```python
from build123d import *

# Parameters (mm, degrees)
BOSS_EXTRUDE1_DEPTH = 10.4
CIRPATTERN1_COUNT   = 10
BOSS_EXTRUDE2_START = 2
SKETCH2_R           = 20
SKETCH2_R_2         = 10.5
BOSS_EXTRUDE2_DEPTH = 2


with BuildPart() as part:
    # Sketch1 → Boss-Extrude1 (new body)
    with BuildSketch(Plane.XY):
        with BuildLine():
            ThreePointArc((9.845402976, 13.551034656), (5.176034656, 15.930196648), (0, 16.75))
            Line((0, 16.75), (1.800167381, 14.035023954))
            ThreePointArc((1.800167381, 14.035023954), (2.401185606, 12.498693353), (3.754556503, 11.555336666))
            ThreePointArc((3.754556503, 11.555336666), (5.403947685, 11.523036823), (6.793214092, 12.412684734))
            Line((6.793214092, 12.412684734), (9.845402976, 13.551034656))
        make_face()
        with BuildLine():
            Line((0, 20), (0, 16.75))
            ThreePointArc((0, 16.75), (5.176034656, 15.930196648), (9.845402976, 13.551034656))
            Line((9.845402976, 13.551034656), (11.755705046, 16.180339887))
            ThreePointArc((11.755705046, 16.180339887), (6.180339887, 19.021130326), (0, 20))
        make_face()
    boss_extrude1 = extrude(amount=BOSS_EXTRUDE1_DEPTH)

    # CirPattern1: Boss-Extrude1 ×10 about axis
    cirpattern1_axis = Axis((0, 0, 0), (0, 0, 1))
    for i in range(1, CIRPATTERN1_COUNT):
        add(boss_extrude1.rotate(cirpattern1_axis, i * 360 / CIRPATTERN1_COUNT))

    # Sketch2 → Boss-Extrude2 (add)
    with BuildSketch(Plane(origin=(0, 0, 0), x_dir=(-1, 0, 0), z_dir=(0, 0, -1)).offset(BOSS_EXTRUDE2_START)):
        Circle(SKETCH2_R)
        Circle(SKETCH2_R_2, mode=Mode.SUBTRACT)
    extrude(amount=-BOSS_EXTRUDE2_DEPTH)


solid = part.part
```
Design review of the part built by this model. Coordinates are the model's own, in mm. A direction names the side the tool comes from. Give positions to 0.01 mm unless a question says otherwise; leave off trailing zeros. Loops run counter-clockwise (first coordinate to the right, second up) from the corner with the lowest first, then second, coordinate; pieces in that order, holes last. Notation, with made-up numbers: M 22.5,-32.5 L 74.5,-32.5 A5 ccw 74.5,-27.5 Z; hole C 85,45.25 d8. An arc over 180 degrees is marked long. Return JSON: item names as keys, results as strings. Group by question number.
Item 1: Insertion check: pin 1 Ø2 at (y, z) = (-14, 4) entering from +X; pin 2 Ø9.5 at (x, y) = (1.5, 2.5) entering from +Z; pin 3 Ø5 at (y, z) = (3, 0) entering from +X; pin 4 Ø1 at (y, z) = (12.5, 5) entering from +X. Each pin has a flat end and moves straight along its axis. Give the tip position at first contact, or say it passes through.
Item 2: Mouldability with a two-part tool opening along X and no side actions: class faces 1 (the flat face through (8.34, -12.99, 5.13)), 2 (the flat face through (-9, -9, -2)) as released by +X, released by -X, zero draft, split by the parting line, or undercut.
Item 3: We need section A-A (y = 1.5). Give the boundary of the cut face in (x, z), and give its area (3 significant figures).
Item 4: For probe 1 along Y at (x, z) = (0, -1.4); probe 2 along Y at (x, z) = (14, 7); probe 3 along Y at (x, z) = (-13, 3.75), list the stretches that pass through material, from the lowest coordinate up.
Item 5: We need section B-B (y = 18.5). Give the boundary of the cut face in (x, z).
Item 6: Tool access review of faces 3 (the flat face through (-0.89, -15.41, 5.13)), 4 (the cylindrical face through (-10, 3.2, -1)): name each direction out of +Z, -Z, +X, -X, +Y, -Y from which nothing blocks a thin tool from reaching the whole face with its end or side.
Output:
{
 "1": {"pin 1": "stops at x = 15.2", "pin 2": "passes through", "pin 3": "stops at x = 19.99", "pin 4": "stops at x = 16"},
 "2": {"face 1": "undercut", "face 2": "zero draft"},
 "3": {"outline": "M -19.94,-2 L -10.39,-2 L -10.39,0 L -12.58,0 L -12.58,10.4 L -19.94,10.4 Z; M 10.39,-2 L 19.94,-2 L 19.94,10.4 L 12.58,10.4 L 12.58,0 L 10.39,0 Z", "area": "191 mm^2"},
 "4": {"probe 1": "y = -20 to -10.5, 10.5 to 20", "probe 2": "y = -14.28 to -5.71, -2.75 to 2.75, 5.71 to 14.28", "probe 3": "y = -15.2 to -5.99, -2.03 to 2.03, 5.99 to 15.2"},
 "5": {"outline": "M -7.6,-2 L 7.6,-2 L 7.6,10.4 L -7.6,10.4 Z"},
 "6": {"face 3": "+Z", "face 4": "+Z, -Z"}
}
